Autodesk Inventor part; units mm, degrees
ref_plane "YZ Plane" through (0, 0, 0) normal (1, 0, 0) x (0, 1, 0)
ref_plane "XZ Plane" through (0, 0, 0) normal (0, 1, 0) x (-1, 0, 0)
ref_plane "XY Plane" through (0, 0, 0) normal (0, 0, 1) x (1, 0, 0)
sketch "Sketch1" plane through (0, 0, 0) normal (0, 1, 0) x (-1, 0, 0)
  line L0 (0, 0) -> (12.192, 0)
  line L1 (12.192, 0) -> (12.192, -12.7)
  line L2 (12.192, -12.7) -> (0, -12.7)
  line L3 (0, -12.7) -> (0, 0)
  line L4 (14.097, -14.605) -> (14.097, 1.905)
  line L5 (14.097, 1.905) -> (-1.905, 1.905)
  line L6 (-1.905, 1.905) -> (-1.905, -14.605)
  line L7 (-1.905, -14.605) -> (14.097, -14.605)
  line L8 (12.192, 0) -> (12.192, 1.905)
  line L9 (0, 0) -> (0, 1.905)
  dimension "d0" = 12.192
  dimension "d1" = 12.7
  dimension "d2" = 1.905
extrude "Extrusion1" add sketch "Sketch1" along normal blind 8.382 contours L3 L2 L1 L8 L5 L4 L7 L6 L9
extrude "Extrusion2" add sketch "Sketch1" against normal blind 1.905
sketch "Sketch2" plane through (0, -1.905, 0) normal (0, -1, 0) x (1, 0, 0)
  circle A0 centre (-6.096, -4.4663) radius 3.7846
  line L0 (-14.097, 1.905) -> (-14.097, -14.605)
  point P0 (0, 0)
  dimension "d7" = 7.5692
  dimension "d8" = 8.001
extrude "Extrusion3" add sketch "Sketch2" along normal blind 1.905
sketch "Sketch3" plane through (1.905, 8.382, -14.605) normal (0, 0, -1) x (-1, 0, 0)
  line L0 (0, 0) -> (16.002, 0)
  line L1 (6.477, 0) -> (9.525, 0)
  line L2 (9.525, 0) -> (9.525, -4.572)
  line L3 (9.525, -4.572) -> (6.477, -4.572)
  line L4 (6.477, -4.572) -> (6.477, 0)
  line L5 (14.097, -8.382) -> (1.905, -8.382)
  line L6 (0, -10.287) -> (0, 0)
  line L7 (1.905, -8.382) -> (1.905, 0)
  dimension "d11" = 3.81
  dimension "d13" = 3.048
  dimension "d14" = 4.572
extrude "Extrusion4" cut sketch "Sketch3" against normal blind 1.905
properties part number "SolenoidHolder"
Model file for the job. Use its own axes, mm. A direction names the side the tool comes from. Round coordinates to 2 decimals unless told otherwise and drop trailing zeros. Loops run counter-clockwise (first coordinate to the right, second up) from the corner with the lowest first, then second, coordinate; pieces in that order, holes last. Notation, with made-up numbers: (41.25, 85.25) - (71.25, 85.25) arc R16 cw to (71.25, 92.25) - close; hole circle Ø6 at (28, 89.25). An arc over 180 degrees is marked (long way). Write each question's results on one line, items separated by ' | '.
(1) Mould opens along X. For faces 1 (the flat face through (-7.62, 6, -14)), 2 (the flat face through (-14.097, 3, -6)), 3 (the flat face through (-6.2, -0.3, 1.905)), 4 (the cylindrical face through (-9.099, -2.844, -2.163)) say: released by +X, released by -X, zero draft, split by the parting line, or undercut.
Answer below:
face 1: undercut | face 2: released by -X | face 3: zero draft | face 4: split by the parting line
(2) 3-axis set-ups, long thin cutter, end or side, ignore diameter. For faces 5 (the flat face through (-6, 3, -14.605)), 6 (the flat face through (0, 4, -5)), 7 (the flat face through (-4, -1.905, -8)), 8 (the flat face through (-6, 3.81, -14)), 9 (the flat face through (-13, 8.382, -8)): which of +Z, -Z, +X, -X, +Y, -Y reach the whole face in a straight line?
Answer below:
face 5: -Z, +X, -X, +Y, -Y | face 6: +Z, +Y | face 7: -Y | face 8: +Z, -Z, +Y | face 9: +Z, -Z, +X, -X, +Y
(3) Wall check: L1, parallel to X at y = 7.5, z = -8 (3 decimals); L2, parallel to Z at x = -8.5, y = 3 (3 decimals); L3, parallel to Y at x = -3, z = -4.5. Give the ranges that are in metal, low to high.
Answer below:
L1: x = -14.097 to -12.192, 0 to 1.905 | L2: z = -14.605 to -12.7 | L3: y = -3.81 to 0
(4) Saw through at A-A, the plane y = 7. List the corners of the cut face in (x, z) (3 decimals), then the cut area to 3 significant figures.
Answer below:
outline: (-14.097, -14.605) - (-7.62, -14.605) - (-7.62, -12.7) - (-12.192, -12.7) - (-12.192, 1.905) - (-14.097, 1.905) - close; (-4.572, -14.605) - (1.905, -14.605) - (1.905, 1.905) - (0, 1.905) - (0, -12.7) - (-4.572, -12.7) - close | area: 80.3 mm^2
(5) Saw through at C-C, the plane y = 1. List the corners of the cut face in (x, z) (3 decimals), then the cut area to 3 significant figures.
Answer below:
outline: (-14.097, -14.605) - (1.905, -14.605) - (1.905, 1.905) - (0, 1.905) - (0, -12.7) - (-12.192, -12.7) - (-12.192, 1.905) - (-14.097, 1.905) - close | area: 86.1 mm^2
(6) Saw through at D-D, the plane x = 0.75. List the corners of the cut face in (y, z) (3 decimals), then the cut area to 3 significant figures.
Answer below:
outline: (-1.905, -14.605) - (8.382, -14.605) - (8.382, 1.905) - (-1.905, 1.905) - close | area: 170 mm^2
(7) Saw through at B-B, the plane z = -13.5. List the corners of the cut face in (x, y) (3 decimals).
Answer below:
outline: (-14.097, -1.905) - (1.905, -1.905) - (1.905, 8.382) - (-4.572, 8.382) - (-4.572, 3.81) - (-7.62, 3.81) - (-7.62, 8.382) - (-14.097, 8.382) - close
(8) Pin check, flat tips, straight feed: pin 1 (2.5 mm diameter, centred on x = -6.5, y = 4.5, fed in from +Z); pin 2 (2 mm diameter, centred on x = -11, z = 0, fed in from +Y); pin 3 (0.6 mm diameter, centred on x = -6.5, z = -14, fed in from +Y). Stop position of each tip, or through.
Answer below:
pin 1: stops at z = -12.7 | pin 2: stops at y = 0 | pin 3: stops at y = 3.81
